```python
from build123d import *

# Parameters (mm, degrees)
EXTRUDE_2_DEPTH     = 25
EXTRUDE_3_DEPTH     = 5
EXTRUDE_5_DEPTH     = 5
SKETCH_8_R          = 1.45
CUT_EXTRUDE_3_DEPTH = 300
SKETCH_9_R          = 1.45
CUT_EXTRUDE_4_DEPTH = 300
SKETCH_10_R         = 2.6
CUT_EXTRUDE_5_DEPTH = 2


with BuildPart() as part:
    # 草图3 → 凸台-拉伸2 (new body)
    with BuildSketch(Plane.XY):
        Polygon((0, 0), (10, 0), (10, 15), (7, 15), (7, 3), (0, 3), align=None)
    extrude(amount=-EXTRUDE_2_DEPTH)

    # 草图4 → 凸台-拉伸3 (add)
    with BuildSketch(Plane.XY):
        Polygon((7, 15), (0, 3), (7, 3), align=None)
    extrude(amount=-EXTRUDE_3_DEPTH)

    # 草图5 → 凸台-拉伸5 (add)
    with BuildSketch(Plane(origin=(0, 0, -25), x_dir=(-1, 0, 0), z_dir=(0, 0, -1))):
        Polygon((-7, 15), (0, 3), (-7, 3), align=None)
    extrude(amount=-EXTRUDE_5_DEPTH)

    # 草图8 → 切除-拉伸3 (cut)
    with BuildSketch(Plane.ZY.offset(-7)):
        with Locations((-16.5, 11.5)):
            Circle(SKETCH_8_R)
        with Locations((-16.5, 6.5)):
            Circle(SKETCH_8_R)
        with Locations((-8.5, 6.5)):
            Circle(SKETCH_8_R)
        with Locations((-8.5, 11.5)):
            Circle(SKETCH_8_R)
    extrude(amount=-CUT_EXTRUDE_3_DEPTH, mode=Mode.SUBTRACT)

    # 草图9 → 切除-拉伸4 (cut)
    with BuildSketch(Plane(origin=(0, 3, 0), x_dir=(1, 0, 0), z_dir=(0, 1, 0))):
        with Locations(Location((3.5, 16.25, 0), (0, 0, 270))):
            Circle(SKETCH_9_R)
        with Locations(Location((3.5, 8.75, 0), (0, 0, 270))):
            Circle(SKETCH_9_R)
    extrude(amount=-CUT_EXTRUDE_4_DEPTH, mode=Mode.SUBTRACT)

    # 草图10 → 切除-拉伸5 (cut)
    with BuildSketch(Plane(origin=(0, 3, 0), x_dir=(1, 0, 0), z_dir=(0, 1, 0))):
        with Locations(Location((3.5, 16.25, 0), (0, 0, 270))):
            Circle(SKETCH_10_R)
        with Locations(Location((3.5, 8.75, 0), (0, 0, 270))):
            Circle(SKETCH_10_R)
    extrude(amount=-CUT_EXTRUDE_5_DEPTH, mode=Mode.SUBTRACT)


solid = part.part
```
Read the model definition and answer for the solid it produces. Units are mm, in the model's axes. A direction names the side the tool comes from. Round coordinates to 2 decimals unless told otherwise and drop trailing zeros. Write each loop counter-clockwise with the first axis right and the second up, starting at its lowest first coordinate (ties: lowest second). Pieces come first, ordered by that corner, then holes. Notation, with made-up numbers: (56, -34) -> (111, -34) arc R16 cw to (111, -20) -> close; hole circle Ø5 at (-10, -3.75). An arc over 180 degrees is marked (long way). Answer in a Markdown table with one row per item. Add a question column.
1) Which of the six approach directions +Z, -Z, +X, -X, +Y, -Y give full straight-line access (tool end or side, diameter ignored) to faces 5 (the face through (7, 9, -12)), 6 (the face through (2.5, 2.01, -13.85)), 7 (the face through (3.56, 0.51, -10.2))?
2) Find section A-A, the plane x = 3.5. Determine the outline of the cut face in (y, z).
3) Given P1, Ø4, axis at x = 3, z = -17, coming from the +Y side; P2, Ø4, axis at y = 10, z = -22.5, coming from the -X side; P3, Ø3.5, axis at x = 3.5, z = -16.25, coming from the +Y side; P4, Ø2.5, axis at y = 11.5, z = -8.5, coming from the -X side, each flat-ended and moving along its own axis, determine where each tip first touches the part or whether it passes through.
4) Find section B-B, the plane y = 7. Determine the outline of the cut face in (x, z).
5) Determine the mould class of faces 1 (the face through (2, 1, -15)), 2 (the face through (10, 7, -12)), 3 (the face through (3.549, 9.084, -2.465)), 4 (the face through (5, 6, -5)) for opening direction X: pulls with the +X half, pulls with the -X half, needs draft (parallel to the pull), parting line crosses it, or undercut.
6) Find section C-C, the plane z = -16.25. Determine the outline of the cut face in (x, y).
7) Consider line 1 (Y direction, x = 8, z = -16.5); line 2 (Z direction, x = 7.5, y = 7); line 3 (Z direction, x = 6, y = 10.75). Determine where each line is inside the solid, lowest interval first.
8) Find section D-D, the plane x = 5.5. Determine the outline of the cut face in (y, z), and give its area (3 significant figures).
Findings below:
| question | item | result |
|---|---|---|
| 1 | face 5 | -X, +Y |
| 1 | face 6 | +Y |
| 1 | face 7 | +Y, -Y |
| 2 | outline | (0, -25) -> (9, -25) -> (9, -20) -> (3, -20) -> (3, -18.85) -> (1, -18.85) -> (1, -17.7) -> (0, -17.7) -> close; (0, -14.8) -> (1, -14.8) -> (1, -13.65) -> (3, -13.65) -> (3, -11.35) -> (1, -11.35) -> (1, -10.2) -> (0, -10.2) -> close; (0, -7.3) -> (1, -7.3) -> (1, -6.15) -> (3, -6.15) -> (3, -5) -> (9, -5) -> (9, 0) -> (0, 0) -> close |
| 3 | P1 | y = 3 |
| 3 | P2 | x = 2.92 |
| 3 | P3 | y = 1 |
| 3 | P4 | through |
| 4 | outline | (2.33, -25) -> (10, -25) -> (10, -17.86) -> (7, -17.86) -> (7, -20) -> (2.33, -20) -> close; (2.33, -5) -> (7, -5) -> (7, -7.14) -> (10, -7.14) -> (10, 0) -> (2.33, 0) -> close; (7, -15.14) -> (10, -15.14) -> (10, -9.86) -> (7, -9.86) -> close |
| 5 | face 1 | undercut |
| 5 | face 2 | pulls with the +X half |
| 5 | face 3 | pulls with the -X half |
| 5 | face 4 | needs draft |
| 6 | outline | (0, 0) -> (2.05, 0) -> (2.05, 1) -> (0.9, 1) -> (0.9, 3) -> (0, 3) -> close; (4.95, 0) -> (10, 0) -> (10, 5.07) -> (7, 5.07) -> (7, 3) -> (6.1, 3) -> (6.1, 1) -> (4.95, 1) -> close; (7, 7.93) -> (10, 7.93) -> (10, 10.07) -> (7, 10.07) -> close; (7, 12.93) -> (10, 12.93) -> (10, 15) -> (7, 15) -> close |
| 7 | line 1 | 0 to 5.05, 7.95 to 10.05, 12.95 to 15 |
| 7 | line 2 | -25 to -17.86, -15.14 to -9.86, -7.14 to 0 |
| 7 | line 3 | -25 to -20, -5 to 0 |
| 8 | outline | (0, -25) -> (12.43, -25) -> (12.43, -20) -> (3, -20) -> (3, -17.91) -> (1, -17.91) -> (1, -14.59) -> (3, -14.59) -> (3, -10.41) -> (1, -10.41) -> (1, -7.09) -> (3, -7.09) -> (3, -5) -> (12.43, -5) -> (12.43, 0) -> (0, 0) -> close |
| 8 | area | 156 mm² |
